from build123d import *

# Parameters (mm, degrees)
BOSS_EXTRUDE3_DEPTH                   = 65
BOSS_EXTRUDE1_DEPTH                   = 6
BOSS_EXTRUDE1_DEPTH_BACK              = 6.25
SKETCH1_5_W                           = 6.6044296
SKETCH1_5_H                           = 19
SKETCH1_5_W_2                         = 10.945657065
BOSS_EXTRUDE2_START                   = -8.75
BOSS_EXTRUDE2_OUTLINE_W               = 40.850086665
BOSS_EXTRUDE2_OUTLINE_H               = 19
BOSS_EXTRUDE2_DEPTH                   = 2.5
REVOLVE2_ANGLE                        = 180
SKETCH1_12_W                          = 10
SKETCH1_12_H                          = 5
REVOLVE4_START                        = -10
REVOLVE4_DEPTH                        = 28.178366994
SERVO_START                           = 67.5
SKETCH9_W                             = 13.671614749
SKETCH9_H                             = 17.273170498
SERVO_WIRE_CUT_DEPTH                  = 18.945657065
CUT_EXTRUDE2_DEPTH                    = 3.5
F_4_0_4_DIAMETER_HOLE1_D              = 4
F_4_0_4_DIAMETER_HOLE1_DEPTH          = 8
F_4_0_4_DIAMETER_HOLE1_CSINK_D        = 5
F_4_0_4_DIAMETER_HOLE1_CSINK_ANGLE    = 90
CIRPATTERN1_COUNT                     = 3
CUT_EXTRUDE4_REACH                    = 151.61
SKETCH21_2_R                          = 4.8
SKETCH12_R                            = 2
HEAT_SET_INSERT_CUT_DEPTH             = 17
HEAT_SET_INSERT_CUT_DIRECTION_2_REACH = 136.816
SKETCH14_R                            = 2
PANEL_HEAT_SET_INSERT_CUT_DEPTH       = 10
BOSS_EXTRUDE10_START                  = -5
SKETCH16_W                            = 7
SKETCH16_H                            = 4.5
BOSS_EXTRUDE10_DEPTH                  = 15
SKETCH18_W                            = 7
SKETCH18_H                            = 3.5
BOSS_EXTRUDE11_DEPTH                  = 10
SKETCH19_R                            = 2
CUT_EXTRUDE1_DEPTH                    = 152.05205452
CHAMFER1_SIZE                         = 2


# Read off the part's stored shape, not the designer's step: Boss-Extrude2, Revolve4
with BuildPart() as part:
    # Sketch4 → Boss-Extrude3 (new body)
    with BuildSketch(Plane.XY):
        Polygon((59.5, -10), (0, -10), (0, -15), (0, -20), (67.5, -20), (67.5, 95.198794821), (0, 95.198794821), (0, 87.198794821), (59.5, 87.198794821), align=None)
    boss_extrude3 = extrude(amount=BOSS_EXTRUDE3_DEPTH)

    # Mirror1: Boss-Extrude3 across plane
    add(boss_extrude3.mirror(Plane(origin=(0, 0, 0), x_dir=(0, 0, 1), z_dir=(1, 0, 0))))

    # Sketch1<5> → Boss-Extrude1 (add, two sides: drawn at the far end of the back side and taken through both)
    with BuildSketch(Plane.XY.offset(-BOSS_EXTRUDE1_DEPTH_BACK)):
        with Locations((21.952128135, -0.5)):
            Rectangle(SKETCH1_5_W, SKETCH1_5_H)
        with Locations((54.027171468, -0.5)):
            Rectangle(SKETCH1_5_W_2, SKETCH1_5_H)
    extrude(amount=BOSS_EXTRUDE1_DEPTH + BOSS_EXTRUDE1_DEPTH_BACK)

    # Boss-Extrude2 outline → Boss-Extrude2 (add)
    with BuildSketch(Plane.XY.offset(BOSS_EXTRUDE2_START)):
        with Locations((39.074956668, -0.5)):
            Rectangle(BOSS_EXTRUDE2_OUTLINE_W, BOSS_EXTRUDE2_OUTLINE_H)
    extrude(amount=BOSS_EXTRUDE2_DEPTH)

    # Sketch1 → Revolve2 (revolve)
    with BuildSketch(Plane.XY):
        Polygon((0, -15), (0, -20), (67.5, -20), (67.5, 95.198794821), (0, 95.198794821), (0, 87.198794821), (59.5, 87.198794821), (59.5, -10), (0, -10), align=None)
    revolve(axis=Axis((0, -1000, 0), (0, 1, 0)), revolution_arc=REVOLVE2_ANGLE)

    # Sketch1<12> → Cut-Revolve4 (revolve, cut)
    with BuildSketch(Plane.XY):
        with Locations((5, -12.5)):
            Rectangle(SKETCH1_12_W, SKETCH1_12_H)
    revolve(axis=Axis((0, -1000, 0), (0, 1, 0)), mode=Mode.SUBTRACT)

    # Revolve4 outline → Revolve4 (add)
    with BuildSketch(Plane(origin=(0, 0, 0), x_dir=(1, 0, 0), z_dir=(0, 1, 0)).offset(REVOLVE4_START)):
        with BuildLine():
            ThreePointArc((-10, 0), (0, 10), (10, 0))
            Line((10, 0), (20, 0))
            ThreePointArc((20, 0), (0, 20), (-20, 0))
            Line((-20, 0), (-10, 0))
        make_face()
    extrude(amount=REVOLVE4_DEPTH)

    # Sketch9 → Servo Wire Cut (cut)
    with BuildSketch(Plane(origin=(0, 0, 0), x_dir=(0, 0, -1), z_dir=(1, 0, 0)).offset(SERVO_START)):
        with Locations((-1.860269854, -12.475825554)):
            Rectangle(SKETCH9_W, SKETCH9_H)
    extrude(amount=-SERVO_WIRE_CUT_DEPTH, mode=Mode.SUBTRACT)

    # Sketch1<13> → Cut-Extrude2 (cut, symmetric)
    with BuildSketch(Plane.XY):
        Polygon((22.754342935, -12.920336749), (59.5, -12.920336749), (59.5, -10), (25.254342935, -10), (25.254342935, 9), (22.754342935, 9), align=None)
    extrude(amount=CUT_EXTRUDE2_DEPTH, both=True, mode=Mode.SUBTRACT)

    # Ø4.0 (4) Diameter Hole1
    with Locations(Plane(origin=(0, 95.198794821, 0), x_dir=(1, 0, 0), z_dir=(0, 1, 0))):
        with Locations((-12.5, 0)):
            f_4_0_4_diameter_hole1 = CounterSinkHole(F_4_0_4_DIAMETER_HOLE1_D / 2, F_4_0_4_DIAMETER_HOLE1_CSINK_D / 2, depth=F_4_0_4_DIAMETER_HOLE1_DEPTH, counter_sink_angle=F_4_0_4_DIAMETER_HOLE1_CSINK_ANGLE)

    # CirPattern1: Ø4.0 (4) Diameter Hole1 ×3 about axis
    cirpattern1_axis = Axis((-27.5, 0, 0), (0, 1, 0))
    for i in range(1, CIRPATTERN1_COUNT):
        add(f_4_0_4_diameter_hole1.rotate(cirpattern1_axis, i * 360 / CIRPATTERN1_COUNT), mode=Mode.SUBTRACT)

    # Sketch21<2> → Cut-Extrude4 (cut, up to next)
    with BuildSketch(Plane(origin=(0, 95.198794821, 0), x_dir=(1, 0, 0), z_dir=(0, 1, 0)), mode=Mode.PRIVATE) as cut_extrude4_sk1:
        with Locations(Location((-27.5, 0, 0), (0, 0, 270))):
            Circle(SKETCH21_2_R)
    cut_extrude4_tool1 = extrude(cut_extrude4_sk1.sketch, amount=-CUT_EXTRUDE4_REACH, mode=Mode.PRIVATE) & part.part
    add(cut_extrude4_tool1.solids().sort_by_distance((-27.5, 95.198795, 0))[0], mode=Mode.SUBTRACT)

    # Sketch12 → Heat Set Insert Cut (cut)
    with BuildSketch(Plane.XY):
        with Locations(Location((54.027171468, 2.884785525, 0), (0, 0, 180))):
            Circle(SKETCH12_R)
        with Locations(Location((15, 2.884785525, 0), (0, 0, 180))):
            Circle(SKETCH12_R)
    extrude(amount=-HEAT_SET_INSERT_CUT_DEPTH, mode=Mode.SUBTRACT)

    # Heat Set Insert Cut direction 2: up to this face of the body (flat: up to its plane)
    heat_set_insert_cut_direction_2_end = Plane(part.part.faces().sort_by_distance((54.027171468, 2.580379847, 6))[0])
    # Sketch12 → Heat Set Insert Cut direction 2 (cut, up to the picked face)
    with BuildSketch(Plane.XY, mode=Mode.PRIVATE) as heat_set_insert_cut_direction_2_sk1:
        with Locations(Location((54.027171468, 2.884785525, 0), (0, 0, 180))):
            Circle(SKETCH12_R)
    heat_set_insert_cut_direction_2_tool1 = split(extrude(heat_set_insert_cut_direction_2_sk1.sketch, amount=HEAT_SET_INSERT_CUT_DIRECTION_2_REACH, mode=Mode.PRIVATE), bisect_by=heat_set_insert_cut_direction_2_end, keep=Keep.BOTH, mode=Mode.PRIVATE)
    # Sketch12 → Heat Set Insert Cut direction 2 (cut, up to the picked face)
    with BuildSketch(Plane.XY, mode=Mode.PRIVATE) as heat_set_insert_cut_direction_2_sk2:
        with Locations(Location((15, 2.884785525, 0), (0, 0, 180))):
            Circle(SKETCH12_R)
    heat_set_insert_cut_direction_2_tool2 = split(extrude(heat_set_insert_cut_direction_2_sk2.sketch, amount=HEAT_SET_INSERT_CUT_DIRECTION_2_REACH, mode=Mode.PRIVATE), bisect_by=heat_set_insert_cut_direction_2_end, keep=Keep.BOTH, mode=Mode.PRIVATE)
    add(heat_set_insert_cut_direction_2_tool1.solids().sort_by(Axis((54.027171, 2.884786, 0), (0, 0, 1)))[0], mode=Mode.SUBTRACT)
    add(heat_set_insert_cut_direction_2_tool2.solids().sort_by(Axis((15, 2.884786, 0), (0, 0, 1)))[0], mode=Mode.SUBTRACT)

    # Sketch14 → Panel Heat Set Insert Cut (cut)
    with BuildSketch(Plane.XY.offset(65)):
        with Locations((-62.379754231, 90.491593885)):
            Circle(SKETCH14_R)
        with Locations((62.379754231, 90.491593885)):
            Circle(SKETCH14_R)
        with Locations((62.379754231, -13.292799065)):
            Circle(SKETCH14_R)
        with Locations((-62.379754231, -13.292799065)):
            Circle(SKETCH14_R)
    extrude(amount=-PANEL_HEAT_SET_INSERT_CUT_DEPTH, mode=Mode.SUBTRACT)

    # Sketch16 → Boss-Extrude10 (add)
    with BuildSketch(Plane.ZY.offset(67.5).offset(BOSS_EXTRUDE10_START)):
        with Locations((-12.283009655, -17.75)):
            Rectangle(SKETCH16_W, SKETCH16_H)
        with Locations((56.5, -17.75)):
            Rectangle(SKETCH16_W, SKETCH16_H)
    boss_extrude10 = extrude(amount=BOSS_EXTRUDE10_DEPTH)

    # Sketch18 → Boss-Extrude11 (add)
    with BuildSketch(Plane(origin=(67.5, 0, 0), x_dir=(0, 0, -1), z_dir=(1, 0, 0))):
        with Locations((-56.5, -18.25)):
            Rectangle(SKETCH18_W, SKETCH18_H)
    extrude(amount=BOSS_EXTRUDE11_DEPTH)

    # Sketch19 → Cut-Extrude1 (cut, through all)
    with BuildSketch(Plane(origin=(0, -15.5, 0), x_dir=(1, 0, 0), z_dir=(0, 1, 0))):
        with Locations(Location((-72.213071965, -56.5, 0), (0, 0, 180))):
            Circle(SKETCH19_R)
        with Locations(Location((-72.213071965, 12.283009655, 0), (0, 0, 180))):
            Circle(SKETCH19_R)
        with Locations(Location((72.5, -56.5, 0), (0, 0, 180))):
            Circle(SKETCH19_R)
    cut_extrude1 = extrude(amount=-CUT_EXTRUDE1_DEPTH, mode=Mode.SUBTRACT)

    # Mirror3: Boss-Extrude10, Cut-Extrude1 across plane
    add(boss_extrude10.mirror(Plane(origin=(0, 0, 0), x_dir=(0, 0, 1), z_dir=(1, 0, 0))))
    add(cut_extrude1.mirror(Plane(origin=(0, 0, 0), x_dir=(0, 0, 1), z_dir=(1, 0, 0))), mode=Mode.SUBTRACT)

    # Chamfer1
    chamfer1_edges = [part.edges().sort_by_distance(p)[0] for p in [
        (0, 95.198794821, -67.5),
        (67.5, 95.198794821, 32.5),
        (-67.5, 95.198794821, 32.5),
    ]]
    chamfer(chamfer1_edges, length=CHAMFER1_SIZE)


solid = part.part
Input: part model. Units: mm. Frame: model coordinates. A direction names the side the tool comes from. Round coordinates to 2 decimals unless told otherwise and drop trailing zeros. Order: outer loops, then holes, each group sorted by start corner. A loop starts at its lowest first (then second) coordinate and runs counter-clockwise, first axis right, second up. Notation, with made-up numbers: (19, 22.25) - (49, 22.25) arc R9 ccw to (49, 31.25) - close; hole circle Ø7 at (51, -34). An arc over 180 degrees is marked (long way). Answer as a JSON object with one key per item and string values. Group by question number.
(1) Cut plane D-D (y = 36). Return loops of the section in (x, z).
(2) Reachability of faces 4 (the face through (-72, -18, -8.783)), 5 (the face through (72, -18, -8.783)), 6 (the face through (-64.378, -13.205, 60.07)) from +Z, -Z, +X, -X, +Y, -Y: full face, straight path, thin tool, end or side. Return the list, or none.
(3) Draft query along Y for faces 1 (the face through (38, 0, -8.75)), 2 (the face through (58, -12, -4.976)), 3 (the face through (74, -15.5, 58)). Return one class per face: released by +Y, released by -Y, zero draft, split by the parting line, or undercut.
(4) Pin query (flat end, axial travel): P1, Ø11, axis at x = 40.5, y = -0.5, coming from the +Z side; P2, Ø5.5, axis at x = 52, y = 3.5, coming from the +Z side; P3, Ø3, axis at x = -15.5, y = 3.5, coming from the +Z side. Return the tip coordinate at first contact, or that it passes through.
(5) Cut plane B-B (z = 25). Return loops of the section in (x, y), then the cut area to 3 significant figures.
(6) Cut plane A-A (y = -7). Return loops of the section in (x, z).
(7) Material intervals for probe 1 along Z at (x, y) = (0, -13.3); probe 2 along Y at (x, z) = (9.5, -30); probe 3 along Z at (x, y) = (-35, 93), sorted ascending. Write a range as from..to.
(8) Cut plane C-C (x = 0). Return loops of the section in (y, z), then the cut area to 3 significant figures.
Here are the results:
{
 "1": {"outline": "(-67.5, 0) arc R67.5 ccw to (67.5, 0) - (67.5, 65) - (59.5, 65) - (59.5, 0) arc R59.5 cw to (-59.5, 0) - (-59.5, 65) - (-67.5, 65) - close"},
 "2": {"face 4": "-X, +Y, -Y", "face 5": "+X, +Y, -Y", "face 6": "+Z"},
 "3": {"face 1": "undercut", "face 2": "zero draft", "face 3": "released by +Y"},
 "4": {"P1": "stops at z = -6.25", "P2": "stops at z = 6", "P3": "stops at z = 0"},
 "5": {"outline": "(-67.5, -20) - (67.5, -20) - (67.5, 93.2) - (65.5, 95.2) - (-65.5, 95.2) - (-67.5, 93.2) - close; hole (-59.5, -10) - (59.5, -10) - (59.5, 87.2) - (-59.5, 87.2) - close", "area": "3,980 mm^2"},
 "6": {"outline": "(-67.5, 0) arc R67.5 ccw to (67.32, -4.98) - (48.55, -4.98) - (48.55, -6.25) - (25.25, -6.25) - (25.25, -3.5) - (22.75, -3.5) - (22.75, 3.5) - (25.25, 3.5) - (25.25, 6) - (18.65, 6) - (18.65, 0) - (10, 0) arc R10 cw to (-10, 0) - (-20, 0) arc R20 ccw to (18.65, -7.22) - (18.65, -8.75) - (58.85, -8.75) arc R59.5 cw to (-59.5, 0) - (-59.5, 65) - (-67.5, 65) - close; (59.5, 8.7) - (67.5, 8.7) - (67.5, 65) - (59.5, 65) - close"},
 "7": {"probe 1": "z = -67.5..-10, 10..65", "probe 2": "y = -20..-10, 87.2..95.2", "probe 3": "z = -57.72..-14.99, -10.99..10.99, 14.99..65"},
 "8": {"outline": "(-20, -67.5) - (93.2, -67.5) - (95.2, -65.5) - (95.2, 65) - (87.2, 65) - (87.2, -59.5) - (-10, -59.5) - (-10, -20) - (18.18, -20) - (18.18, -10) - (-15, -10) - (-15, 10) - (-10, 10) - (-10, 65) - (-20, 65) - close", "area": "3,340 mm^2"}
}
